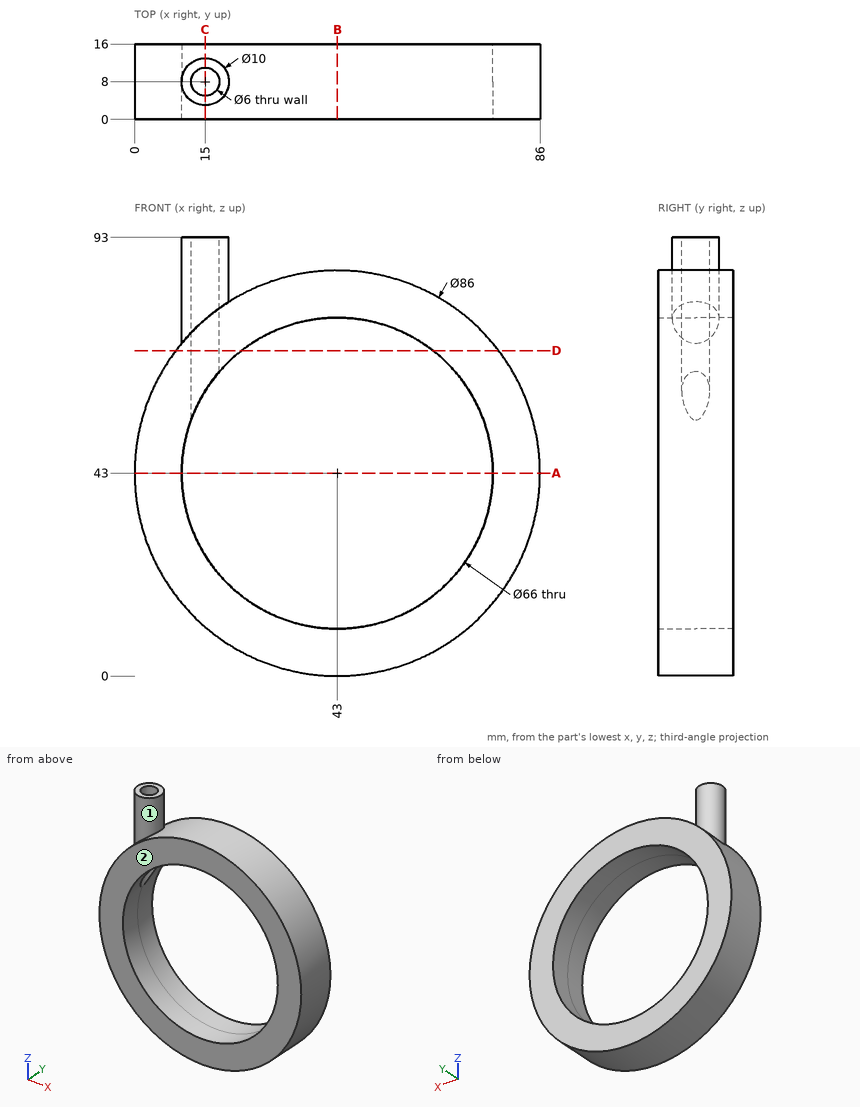
Job drawing, mm, ordinate dimensions from the low corner. One solid piece. Give positions to 0.01 mm unless a question says otherwise; leave off trailing zeros. Loops run counter-clockwise (first coordinate to the right, second up) from the corner with the lowest first, then second, coordinate; pieces in that order, holes last. Notation, with made-up numbers: M 36.5,37.25 L 42.5,37.25 A19 cw 42.5,47.25 Z; hole C -29.5,32 d2. An arc over 180 degrees is marked long. Put each result on its own line as item: value. Start each with the question number.
1) Saw through at D-D (z = 69). List the corners of the cut face in (x, y), then the cut area to 3 significant figures.
2) Pull direction X, two halves, no side cores. Call the marked faces 1 and 2: +X half, -X half, draft (parallel to the pull), parting line (faces both ways), or undercut.
3) Flat gauge pins, fed straight in: pin 1 (2 mm diameter, centred on y = 10.5, z = 46.5, fed in from -X); pin 2 (2 mm diameter, centred on x = 45, y = 7.5, fed in from -Z); pin 3 (1 mm diameter, centred on x = 40, y = 4.5, fed in from +Z); pin 4 (8 mm diameter, centred on x = 19.5, z = 52, fed in from -Y). Where does each tip first touch, or does it go through?
4) Saw through at B-B (x = 43). List the corners of the cut face in (y, z), then the cut area to 3 significant figures.
5) Saw through at C-C (x = 15). List the corners of the cut face in (y, z).
6) Probe probe 1 along Z at (x, y) = (43, 12); probe 2 along Y at (x, z) = (15, 79); probe 3 along Y at (x, z) = (15, 74.5). List the from-to ranges inside material, lowest first.
7) Saw through at A-A (z = 43). List the corners of the cut face in (x, y), then the cut area to 3 significant figures.
Numbers:
1. outline: M 8.75,0 L 22.68,0 L 22.68,16 L 8.75,16 Z; M 63.32,0 L 77.25,0 L 77.25,16 L 63.32,16 Z; hole C 15,8 d6
1. area: 417 mm^2
2. face 1: undercut
2. face 2: draft
3. pin 1: x = 0.07
3. pin 2: z = 0.01
3. pin 3: z = 85.93
3. pin 4: through
4. outline: M 0,0 L 16,0 L 16,10 L 0,10 Z; M 0,76 L 16,76 L 16,86 L 0,86 Z
4. area: 320 mm^2
5. outline: M 0,10.37 L 16,10.37 L 16,25.54 L 0,25.54 Z; M 0,60.46 L 5,60.46 L 5,93 L 3,93 L 3,75.63 L 0,75.63 Z; M 11,60.46 L 16,60.46 L 16,75.63 L 13,75.63 L 13,93 L 11,93 Z
6. probe 1: 0 to 10, 76 to 86
6. probe 2: 3 to 5, 11 to 13
6. probe 3: 0 to 5, 11 to 16
7. outline: M 0,0 L 10,0 L 10,16 L 0,16 Z; M 76,0 L 86,0 L 86,16 L 76,16 Z
7. area: 320 mm^2
